from build123d import *

# Parameters (mm, degrees)
F1_DEPTH = 12.7
F2_DEPTH = 6.35
F4_DEPTH = 19.051
F5_R     = 5.08


# Not quite as in the source:
# - a feature names something its author has since deleted; it is built from what else it names


with BuildPart() as f1:
    # F0 (on Top) → F1 (new body, symmetric)
    with BuildSketch(Plane.XY):
        Polygon((0.2673684239, -2.5617282353), (-12.7, -2.5617282353), (-25.4, -2.5617282353), (-25.4, -15.2617282353), (25.4, -15.2617282353), (25.4, -2.5617282353), (12.7, -2.5617282353), align=None)
    extrude(amount=F1_DEPTH, both=True)

    # F0 (on Top) → F2 (join, symmetric)
    with BuildSketch(Plane.XY):
        Polygon((6.35, 8.4367943928), (0.2673684239, -2.5617282353), (12.7, -2.5617282353), align=None)
        Polygon((-6.35, 8.4367943928), (-12.7, -2.5617282353), (0.2673684239, -2.5617282353), align=None)
        Polygon((0, 19.4353170208), (-6.35, 8.4367943928), (6.35, 8.4367943928), align=None)
        Polygon((-6.35, 8.4367943928), (0.2673684239, -2.5617282353), (6.35, 8.4367943928), align=None)
    extrude(amount=F2_DEPTH, both=True)

    # F3 (on face) → F4 (cut, through all)
    with BuildSketch(Plane.XY.offset(6.35)):
        Polygon((5.4885434949, 7.9287943928), (-5.4514978916, 7.9287943928), (0.2488394649, -1.5455593664), align=None)
    extrude(amount=-F4_DEPTH, mode=Mode.SUBTRACT)

    # F5
    f5_edges = [f1.edges().sort_by_distance(p)[0] for p in [
        (-25.4, -8.911728, 12.7),
        (-25.4, -8.911728, -12.7),
        (25.4, -8.911728, -12.7),
        (25.4, -8.911728, 12.7),
        (-25.4, -15.261728, 0),
        (0, -15.261728, -12.7),
        (25.4, -15.261728, 0),
        (0, -15.261728, 12.7),
        (0, -2.561728, 12.7),
        (0, -2.561728, -12.7),
        (25.4, -2.561728, 0),
        (-25.4, -2.561728, 0),
    ]]
    fillet(f5_edges, radius=F5_R)


solid = f1.part
Geometry: final body of the model. Coordinates: model frame, mm. A direction names the side the tool comes from. Coordinates: 2 decimals unless noted, no trailing zeros. Order: outer loops, then holes, each group sorted by start corner. A loop starts at its lowest first (then second) coordinate and runs counter-clockwise, first axis right, second up.
(1) Material intervals for probe 1 along Y at (x, z) = (4, -6.25); probe 2 along Y at (x, z) = (-13, 6.5); probe 3 along Y at (x, z) = (-4, -4), sorted ascending.
(2) Section query A-A (y = -9). Return the cut outline in (x, z).
(3) Section query D-D (x = 16.5). Return the cut outline in (y, z).
(4) Section query B-B (z = -5.5). Return the cut outline in (x, y).
(5) Draft query along Y for faces 6 (the face through (-0.28, -4.09, -11.25)), 7 (the face through (23.872, -8.894, -11.251)), 8 (the face through (2.832, 3.125, 0.089)), 9 (the face through (23.872, -13.813, 0.107)). Return one class per face: pulls with the +Y half, pulls with the -Y half, needs draft (parallel to the pull), parting line crosses it, or undercut.
(6) First-contact query: pin 1 (10 mm diameter, centred on x = -4.5, y = 12, fed in from +Z); pin 2 (3 mm diameter, centred on x = 14, z = 8.5, fed in from +Y); pin 3 (8 mm diameter, centred on x = -3.5, y = 13, fed in from -Z). Flat tips, straight axial feed; report the tip coordinate or a pass-through.
(7) Access query for faces 1 (the face through (0, 7.929, 0)), 2 (the face through (0, 9, -6.35)), 3 (the face through (0, 9, 6.35)), 4 (the face through (-23.951, -8.93, 11.172)), 5 (the face through (23.872, -8.894, 11.251)). Directions: +Z, -Z, +X, -X, +Y, -Y. A direction counts if a zero-diameter tool reaches every point of the face in a straight line with its end or side. Return the directions, or none.
(8) Section query C-C (y = 1.5). Return the cut outline in (x, z), plus the area to 3 significant figures.
Solution:
1. probe 1: y = -15.26 to 5.24, 7.93 to 12.51
1. probe 2: y = -15.26 to -2.56
1. probe 3: y = -15.26 to 5.52, 7.93 to 12.51
2. outline: (-25.4, -7.62) arc R5.08 ccw to (-20.32, -12.7) - (20.32, -12.7) arc R5.08 ccw to (25.4, -7.62) - (25.4, 7.62) arc R5.08 ccw to (20.32, 12.7) - (-20.32, 12.7) arc R5.08 ccw to (-25.4, 7.62) - close
3. outline: (-15.26, -7.62) arc R5.08 ccw to (-10.18, -12.7) - (-7.64, -12.7) arc R5.08 ccw to (-2.56, -7.62) - (-2.56, 7.62) arc R5.08 ccw to (-7.64, 12.7) - (-10.18, 12.7) arc R5.08 ccw to (-15.26, 7.62) - close
4. outline: (-25.4, -10.18) arc R5.08 ccw to (-20.32, -15.26) - (20.32, -15.26) arc R5.08 ccw to (25.4, -10.18) - (25.4, -7.64) arc R5.08 ccw to (20.32, -2.56) - (12.7, -2.56) - (0, 19.44) - (-12.7, -2.56) - (-20.32, -2.56) arc R5.08 ccw to (-25.4, -7.64) - close; hole (-5.45, 7.93) - (0.25, -1.55) - (5.49, 7.93) - close
5. face 6: pulls with the +Y half
5. face 7: needs draft
5. face 8: undercut
5. face 9: pulls with the -Y half
6. pin 1: stops at z = 6.35
6. pin 2: stops at y = -2.56
6. pin 3: stops at z = -6.35
7. face 1: +Z, -Z
7. face 2: -Z, +X, -X, +Y
7. face 3: +Z, +X, -X, +Y
7. face 4: +Z, -X, +Y, -Y
7. face 5: +Z, +X, +Y, -Y
8. outline: (-10.35, -6.35) - (-1.58, -6.35) - (-1.58, 6.35) - (-10.35, 6.35) - close; (1.93, -6.35) - (10.35, -6.35) - (10.35, 6.35) - (1.93, 6.35) - close
8. area: 218 mm2
